The listing builds one solid part. Answer for the finished solid, in the listing's coordinates (mm). Face numbers are marked on the shaded views. A direction names the side the tool comes from. Coordinates: 2 decimals unless noted, no trailing zeros. Order: outer loops, then holes, each group sorted by start corner. A loop starts at its lowest first (then second) coordinate and runs counter-clockwise, first axis right, second up. Notation, with made-up numbers: (18.25, 47.5) -> (65.25, 47.5) arc R11 ccw to (65.25, 67.5) -> close; hole circle Ø2 at (31, 81.25). An arc over 180 degrees is marked (long way). Write each question's results on one line, items separated by ' | '. Start each with the question number.
(1) The part is cut by section A-A, the plane x = 0. Give the vertices of the cut face in (y, z), then the cut area to 3 significant figures.
(2) Given pin 1 (4 mm diameter, centred on x = 0, z = 0, fed in from -Y), flat-ended and moving along its own axis, determine where the tip first touches the part or whether it passes through.
(3) A tool of negligible diameter and unlimited length cuts with its end or side. For the marked faces 5 and 6, from which of +Z, -Z, +X, -X, +Y, -Y can it reach the whole face along a straight path? Write none if from no direction.
(4) Determine the mould class of the marked faces 1, 2, 3 and 4 for opening direction Z: +Z half, -Z half, draft (parallel to the pull), parting line (faces both ways), or undercut.
(5) Straight lines are drawn through the part: L1, parallel to X at y = 4.6, z = 0; L2, parallel to Y at x = -3, z = -0.5; L3, parallel to Z at x = 2.5, y = -3.5. For each, find the intervals that lie inside material, in ascending order.
(6) The part is cut by section D-D, the plane y = -2.5. Give the vertices of the cut face in (x, z).
(7) The part is cut by section C-C, the plane x = 3. Give the vertices of the cut face in (y, z).
(8) The part is cut by section B-B, the plane z = 3. Give the vertices of the cut face in (x, y), then the cut area to 3 significant figures.
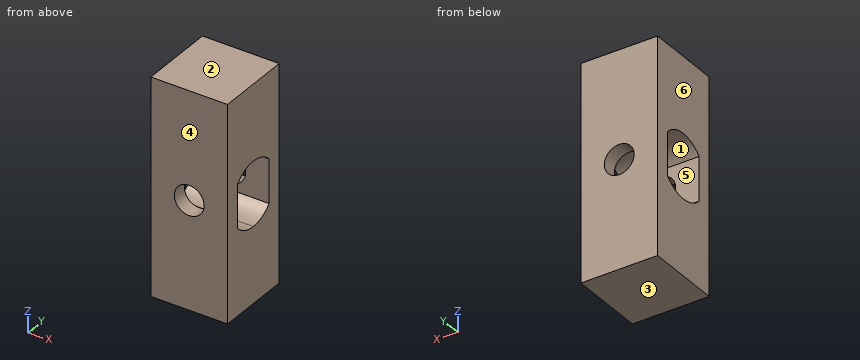
```python
from build123d import *

# Parameters (mm, degrees)
SKETCH1_W           = 12.446
SKETCH1_H           = 12.446
BOSS_EXTRUDE1_DEPTH = 17.4625
SKETCH2_W           = 7.098379816
SKETCH2_H           = 7.62
CUT_EXTRUDE1_DEPTH  = 23.328626273
SKETCH3_R           = 2.413
CUT_EXTRUDE2_DEPTH  = 23.328626273


with BuildPart() as part:
    # Sketch1 → Boss-Extrude1 (new, symmetric)
    with BuildSketch(Plane.XY):
        Rectangle(SKETCH1_W, SKETCH1_H)
    extrude(amount=BOSS_EXTRUDE1_DEPTH, both=True)

    # Sketch2 → Cut-Extrude1 (cut, through all)
    with BuildSketch(Plane(origin=(6.223, 0, 0), x_dir=(0, 0, -1), z_dir=(1, 0, 0))):
        with BuildLine():
            ThreePointArc((-3.549189908, 3.81), (-5.207, 0), (-3.549189908, -3.81))
            Line((-3.549189908, -3.81), (-3.549189908, 3.81))
        make_face()
        Rectangle(SKETCH2_W, SKETCH2_H)
        with BuildLine():
            Line((3.549189908, 3.81), (3.549189908, -3.81))
            ThreePointArc((3.549189908, -3.81), (4.774593221, -2.077524627), (5.207, 0))
            ThreePointArc((5.207, 0), (4.774593221, 2.077524627), (3.549189908, 3.81))
        make_face()
    extrude(amount=-CUT_EXTRUDE1_DEPTH, mode=Mode.SUBTRACT)

    # Sketch3 → Cut-Extrude2 (cut, through all)
    with BuildSketch(Plane(origin=(0, 6.223, 0), x_dir=(1, 0, 0), z_dir=(0, 1, 0))):
        with Locations(Location((0, 0, 0), (0, 0, 270))):
            Circle(SKETCH3_R)
    extrude(amount=-CUT_EXTRUDE2_DEPTH, mode=Mode.SUBTRACT)


solid = part.part
```
Established:
1) outline: (-6.22, -17.46) -> (6.22, -17.46) -> (6.22, -2.41) -> (3.81, -2.41) -> (3.81, -3.55) arc R5.21 cw to (-3.81, -3.55) -> (-3.81, -2.41) -> (-6.22, -2.41) -> close; (-6.22, 2.41) -> (-3.81, 2.41) -> (-3.81, 3.55) arc R5.21 cw to (3.81, 3.55) -> (3.81, 2.41) -> (6.22, 2.41) -> (6.22, 17.46) -> (-6.22, 17.46) -> close | area: 340 mm^2
2) pin 1: passes through
3) face 5: +X, -X | face 6: +Z, -Z, -X, +Y, -Y
4) face 1: undercut | face 2: +Z half | face 3: -Z half | face 4: draft
5) L1: x = -6.22 to -2.41, 2.41 to 6.22 | L2: y = -6.22 to -3.81, 3.81 to 6.22 | L3: z = -17.46 to -3.86, 3.86 to 17.46
6) outline: (-6.22, -17.46) -> (6.22, -17.46) -> (6.22, -4.57) -> (-6.22, -4.57) -> close; (-6.22, 4.57) -> (6.22, 4.57) -> (6.22, 17.46) -> (-6.22, 17.46) -> close
7) outline: (-6.22, -17.46) -> (6.22, -17.46) -> (6.22, 17.46) -> (-6.22, 17.46) -> close; hole (-3.81, -3.55) arc R5.21 ccw to (3.81, -3.55) -> (3.81, 3.55) arc R5.21 ccw to (-3.81, 3.55) -> close
8) outline: (-6.22, -6.22) -> (6.22, -6.22) -> (6.22, -3.81) -> (-6.22, -3.81) -> close; (-6.22, 3.81) -> (6.22, 3.81) -> (6.22, 6.22) -> (-6.22, 6.22) -> close | area: 60.1 mm^2
